Source: three-view drawing plus pictorial views. Frame: mm from the lowest corner of the part. Round coordinates to 2 decimals unless told otherwise and drop trailing zeros. Order: outer loops, then holes, each group sorted by start corner. A loop starts at its lowest first (then second) coordinate and runs counter-clockwise, first axis right, second up. Notation, with made-up numbers: (72.5, 9.25) - (123.5, 9.25) arc R31 cw to (123.5, 35.25) - close; hole circle Ø4 at (-26, -13). An arc over 180 degrees is marked (long way). One line per item, written item: value. Start each with the question number.
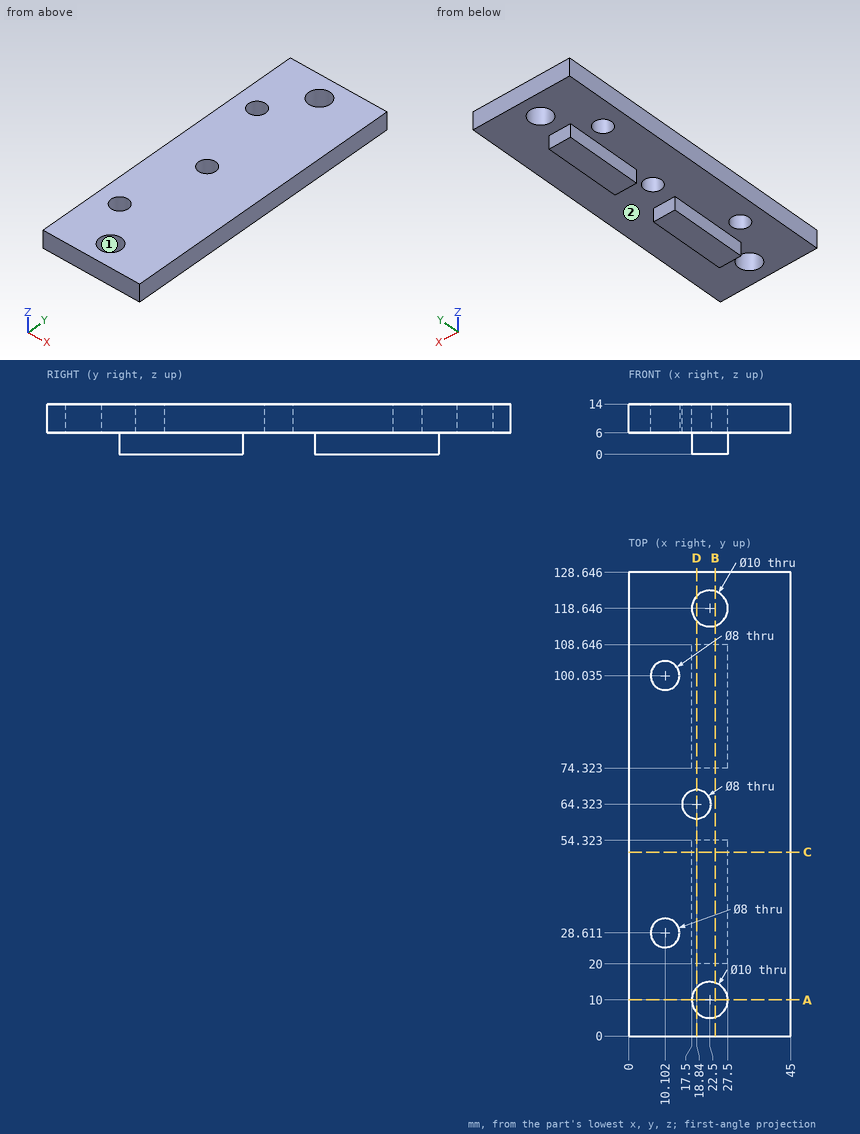
Item 1: Section query B-B on x = 24. Return loops of the section in (y, z) (1 decimal).
Item 2: First-contact query: pin 1 Ø6.5 at (y, z) = (95, 2.5) entering from -X; pin 2 Ø1.8 at (x, z) = (24.5, 1.5) entering from -Y; pin 3 Ø12 at (x, y) = (35.5, 18.5) entering from -Z; pin 4 Ø13.5 at (x, y) = (21, 60.5) entering from -Z. Flat tips, straight axial feed; report the tip coordinate or a pass-through.
Item 3: Section query C-C on y = 51. Return loops of the section in (x, z).
Item 4: Section query A-A on y = 10. Return loops of the section in (x, z), and give its area (3 significant figures).
Item 5: Line query: L1, parallel to Y at x = 26, z = 9.5 (1 decimal); L2, parallel to X at y = 10, z = 11.5; L3, parallel to X at y = 40.5, z = 4. Output: solid intervals per line, ascending.
Item 6: Pull-direction query (X, two-part tool) for the marked faces 1 and 2; classes: released by +X, released by -X, zero draft, split by the parting line, or undercut.
Item 7: Section query D-D on x = 18.84. Return loops of the section in (y, z), and give its area (3 significant figures).
Geometry results:
1. outline: (0, 6) - (5.2, 6) - (5.2, 14) - (0, 14) - close; (14.8, 6) - (20, 6) - (20, 0) - (54.3, 0) - (54.3, 6) - (74.3, 6) - (74.3, 0) - (108.6, 0) - (108.6, 6) - (113.9, 6) - (113.9, 14) - (14.8, 14) - close; (123.4, 6) - (128.6, 6) - (128.6, 14) - (123.4, 14) - close
2. pin 1: stops at x = 17.5
2. pin 2: stops at y = 20
2. pin 3: stops at z = 6
2. pin 4: stops at z = 0
3. outline: (0, 6) - (17.5, 6) - (17.5, 0) - (27.5, 0) - (27.5, 6) - (45, 6) - (45, 14) - (0, 14) - close
4. outline: (0, 6) - (17.5, 6) - (17.5, 14) - (0, 14) - close; (27.5, 6) - (45, 6) - (45, 14) - (27.5, 14) - close
4. area: 280 mm^2
5. L1: y = 0 to 6.4, 13.6 to 115.1, 122.2 to 128.6
5. L2: x = 0 to 17.5, 27.5 to 45
5. L3: x = 17.5 to 27.5
6. face 1: undercut
6. face 2: zero draft
7. outline: (0, 6) - (6.59, 6) - (6.59, 14) - (0, 14) - close; (13.41, 6) - (20, 6) - (20, 0) - (54.32, 0) - (54.32, 6) - (60.32, 6) - (60.32, 14) - (13.41, 14) - close; (68.32, 6) - (74.32, 6) - (74.32, 0) - (108.65, 0) - (108.65, 6) - (115.24, 6) - (115.24, 14) - (68.32, 14) - close; (122.05, 6) - (128.65, 6) - (128.65, 14) - (122.05, 14) - close
7. area: 1,270 mm^2
